Check sheet for the modelled part. Datum: model origin and axes. Units: mm. Face numbers are marked on the shaded views. Give positions to 0.01 mm unless a question says otherwise; leave off trailing zeros. Order: outer loops, then holes, each group sorted by start corner. A loop starts at its lowest first (then second) coordinate and runs counter-clockwise, first axis right, second up.
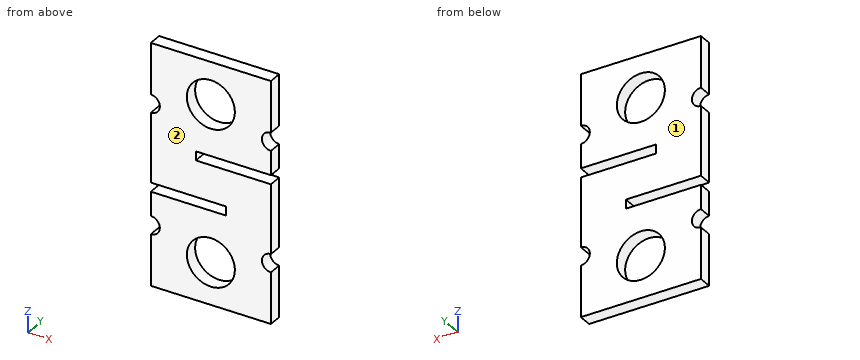
from build123d import *

# Parameters (mm, degrees)
CROQUIS1_R              = 8
SALIENTE_EXTRUIR1_DEPTH = 4.45


with BuildPart() as part:
    # Croquis1 → Saliente-Extruir1 (new body)
    with BuildSketch(Plane(origin=(0, 0, 0), x_dir=(1, 0, 0), z_dir=(0, 1, 0))):
        with BuildLine():
            Line((-20, -41.25), (20, -41.25))
            Line((20, -41.25), (20, -24.25))
            ThreePointArc((20, -24.25), (17, -21.25), (20, -18.25))
            Line((20, -18.25), (20, -10.25))
            Line((20, -10.25), (-5, -10.25))
            Line((-5, -10.25), (-5, -7.25))
            Line((-5, -7.25), (20, -7.25))
            Line((20, -7.25), (20, 15.75))
            ThreePointArc((20, 15.75), (17, 18.75), (20, 21.75))
            Line((20, 21.75), (20, 38.75))
            Line((20, 38.75), (-20, 38.75))
            Line((-20, 38.75), (-20, 21.75))
            ThreePointArc((-20, 21.75), (-17, 18.75), (-20, 15.75))
            Line((-20, 15.75), (-20, 7.75))
            Line((-20, 7.75), (5, 7.75))
            Line((5, 7.75), (5, 4.75))
            Line((5, 4.75), (-20, 4.75))
            Line((-20, 4.75), (-20, -18.25))
            ThreePointArc((-20, -18.25), (-17, -21.25), (-20, -24.25))
            Line((-20, -24.25), (-20, -41.25))
        make_face()
        with Locations((0, -27.25)):
            Circle(CROQUIS1_R, mode=Mode.SUBTRACT)
        with Locations((0, 24.75)):
            Circle(CROQUIS1_R, mode=Mode.SUBTRACT)
    extrude(amount=SALIENTE_EXTRUIR1_DEPTH)


solid = part.part
1) Section check D-D, the plane x = -15.5. Record the cut outline in (y, z), then the cut area to 3 significant figures.
Recorded:
outline: (0, -38.75) - (4.45, -38.75) - (4.45, -7.75) - (0, -7.75) - close; (0, -4.75) - (4.45, -4.75) - (4.45, 41.25) - (0, 41.25) - close
area: 343 mm2
2) Section check A-A, the plane x = 0. Record the cut outline in (y, z).
Recorded:
outline: (0, -38.75) - (4.45, -38.75) - (4.45, -32.75) - (0, -32.75) - close; (0, -16.75) - (4.45, -16.75) - (4.45, -7.75) - (0, -7.75) - close; (0, -4.75) - (4.45, -4.75) - (4.45, 7.25) - (0, 7.25) - close; (0, 10.25) - (4.45, 10.25) - (4.45, 19.25) - (0, 19.25) - close; (0, 35.25) - (4.45, 35.25) - (4.45, 41.25) - (0, 41.25) - close
3) Section check C-C, the plane y = 1.7. Record the cut outline in (x, z).
Recorded:
outline: (-20, -38.75) - (20, -38.75) - (20, -21.75) arc R3 cw to (20, -15.75) - (20, 7.25) - (-5, 7.25) - (-5, 10.25) - (20, 10.25) - (20, 18.25) arc R3 cw to (20, 24.25) - (20, 41.25) - (-20, 41.25) - (-20, 24.25) arc R3 cw to (-20, 18.25) - (-20, -4.75) - (5, -4.75) - (5, -7.75) - (-20, -7.75) - (-20, -15.75) arc R3 cw to (-20, -21.75) - close; hole circle Ø16 at (0, -24.75); hole circle Ø16 at (0, 27.25)
4) Depth check by flat-ended pin: pin 1 Ø1.5 at (y, z) = (2, 8.5) entering from +X. Enter the tip coordinate at first touch or a pass-through.
Recorded:
pin 1: stops at x = -5
5) Material ranges on L1, parallel to Z at x = 0, y = 3.15; L2, parallel to Z at x = -9, y = 1.4; L3, parallel to X at y = 1.4, z = 27.25, recorded low to high.
Recorded:
L1: z = -38.75 to -32.75, -16.75 to -7.75, -4.75 to 7.25, 10.25 to 19.25, 35.25 to 41.25
L2: z = -38.75 to -7.75, -4.75 to 41.25
L3: x = -20 to -8, 8 to 20
6) Section check B-B, the plane z = 27.25. Record the cut outline in (x, y).
Recorded:
outline: (-20, 0) - (-8, 0) - (-8, 4.45) - (-20, 4.45) - close; (8, 0) - (20, 0) - (20, 4.45) - (8, 4.45) - close
7) Draft check along Y on the marked faces 1 and 2. Enter one of: +Y half, -Y half, draft (parallel to the pull), parting line (faces both ways), or undercut.
Recorded:
face 1: +Y half
face 2: -Y half
